Model file for the job. Use its own axes, mm. Round coordinates to 2 decimals unless told otherwise and drop trailing zeros. Order: outer loops, then holes, each group sorted by start corner. A loop starts at its lowest first (then second) coordinate and runs counter-clockwise, first axis right, second up. Notation, with made-up numbers: M 79.5,-19.75 L 134.5,-19.75 A10 ccw 134.5,-2.75 Z; hole C 5.25,-11 d4. An arc over 180 degrees is marked long. Return JSON: item names as keys, results as strings. Group by question number.
Item 1: Slice it at B-B on y = 6.5. Write the cut outline in (x, z).
Item 2: Pin check, flat tips, straight feed: pin 1 Ø3 at (x, z) = (63.5, 0) entering from +Y; pin 2 Ø2 at (y, z) = (7.5, 3) entering from +X; pin 3 Ø6.5 at (x, z) = (-63.5, 0) entering from -Y; pin 4 Ø2 at (y, z) = (6, -1.5) entering from +X. Stop position of each tip, or through.
Item 3: Probe line 1 along X through (y, z) = (8.5, 0); line 2 along Z through (x, y) = (63.5, 5.75); line 3 along X through (y, z) = (10, -1). List the from-to ranges inside material, lowest first.
Item 4: Slice it at A-A on z = 0. Write the cut outline in (x, y), then the cut area to 3 significant figures.
Item 5: Slice it at C-C on z = -5.5. Write the cut outline in (x, y).
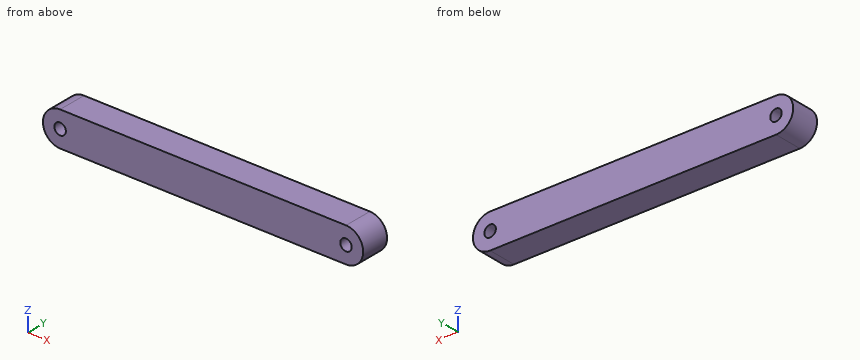
from build123d import *

# Parameters (mm, degrees)
BOSS_EXTRUDE1_DEPTH = 12.7
SKETCH4_R           = 2.54
CUT_EXTRUDE3_DEPTH  = 73.645776202


with BuildPart() as part:
    # Sketch3 → Boss-Extrude1 (new body)
    with BuildSketch(Plane(origin=(0, 0, 0), x_dir=(1, 0, 0), z_dir=(0, 1, 0))):
        with BuildLine():
            Line((-63.5, 7.62), (63.5, 7.62))
            ThreePointArc((63.5, 7.62), (71.12, 0), (63.5, -7.62))
            Line((63.5, -7.62), (-63.5, -7.62))
            ThreePointArc((-63.5, -7.62), (-71.12, 0), (-63.5, 7.62))
        make_face()
    extrude(amount=BOSS_EXTRUDE1_DEPTH)

    # Sketch4 → Cut-Extrude3 (cut, through all)
    with BuildSketch(Plane(origin=(0, 12.7, 0), x_dir=(1, 0, 0), z_dir=(0, 1, 0))):
        with Locations(Location((-63.5, 0, 0), (0, 0, 270))):
            Circle(SKETCH4_R)
        with Locations(Location((63.5, 0, 0), (0, 0, 90))):
            Circle(SKETCH4_R)
    extrude(amount=-CUT_EXTRUDE3_DEPTH, mode=Mode.SUBTRACT)


solid = part.part
Output values:
{
 "1": {"outline": "M -63.5,-7.62 L 63.5,-7.62 A7.62 ccw 63.5,7.62 L -63.5,7.62 A7.62 ccw Z; hole C -63.5,0 d5.08; hole C 63.5,0 d5.08"},
 "2": {"pin 1": "through", "pin 2": "x = 70.85", "pin 3": "y = 0", "pin 4": "x = 71.1"},
 "3": {"line 1": "-71.12 to -66.04, -60.96 to 60.96, 66.04 to 71.12", "line 2": "-7.62 to -2.54, 2.54 to 7.62", "line 3": "-71.05 to -65.83, -61.17 to 61.17, 65.83 to 71.05"},
 "4": {"outline": "M -71.12,0 L -66.04,0 L -66.04,12.7 L -71.12,12.7 Z; M -60.96,0 L 60.96,0 L 60.96,12.7 L -60.96,12.7 Z; M 66.04,0 L 71.12,0 L 71.12,12.7 L 66.04,12.7 Z", "area": "1,680 mm²"},
 "5": {"outline": "M -68.77,0 L 68.77,0 L 68.77,12.7 L -68.77,12.7 Z"}
}
